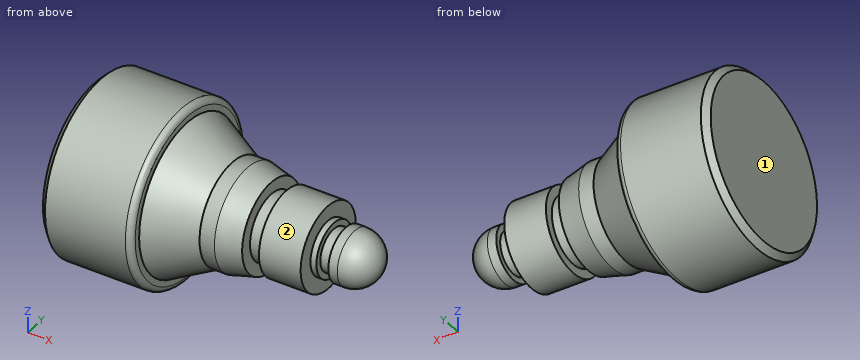
from build123d import *

# Parameters (mm, degrees)
F2_SIZE = 2
F3_R    = 2
F4_R    = 9


with BuildPart() as f1:
    # F0 (on Front) → F1 (revolve)
    with BuildSketch(Plane.XZ):
        Polygon((0, 29), (0, 0), (96, 0), (96, 9), (84, 9), (84, 7), (80, 7), (80, 9), (78, 9), (78, 14), (64, 14), (64, 11), (59, 11), (59, 15), (51, 17), (46, 17), (31, 25), (31, 29), align=None)
    revolve(axis=Axis((48, 0, 0), (1, 0, 0)))

    # F2
    f2_edges = [f1.edges().sort_by_distance(p)[0] for p in [
        (0, 0, -29),
    ]]
    chamfer(f2_edges, length=F2_SIZE)

    # F3
    f3_edges = [f1.edges().sort_by_distance(p)[0] for p in [
        (31, 0, -29),
    ]]
    fillet(f3_edges, radius=F3_R)

    # F4
    f4_edges = [f1.edges().sort_by_distance(p)[0] for p in [
        (96, 0, -9),
    ]]
    fillet(f4_edges, radius=F4_R)


solid = f1.part
Verification items for the finished model (mm, model axes). Face numbers are marked on the shaded views. A direction names the side the tool comes from. Coordinates: 2 decimals unless noted, no trailing zeros. Order: outer loops, then holes, each group sorted by start corner. A loop starts at its lowest first (then second) coordinate and runs counter-clockwise, first axis right, second up. Notation, with made-up numbers: M 18,-28.75 L 28,-28.75 A20 cw 28,6.25 Z; hole C 1.25,36 d1. An arc over 180 degrees is marked long. One line per item, written item: value. Start each with the question number.
Item 1: Access from +Z, -Z, +X, -X, +Y, -Y to the whole of each face (thin tool, end or side, straight path). Record for the marked faces 1 and 2.
Item 2: Scan lines: probe 1 along X at (y, z) = (-10.5, 2.5); probe 2 along Y at (x, z) = (11, 23.5); probe 3 along X at (y, z) = (-25, -8). Record each from-to range of solid material in increasing order.
Item 3: Gauge pin test, flat ends, axial feed: pin 1 (5 mm diameter, centred on y = 19.5, z = -1, fed in from -X); pin 2 (10 mm diameter, centred on x = 73.5, y = -12, fed in from +Z); pin 3 (1 mm diameter, centred on x = 17.5, z = 16.5, fed in from +Y); pin 4 (3 mm diameter, centred on y = -12.5, z = 1, fed in from +X). Record the tip position at first contact, or that the pin passes through.
Item 4: Sectioned sample at A-A (x = 71). Enter the section's corners in (y, z).
Conclusion:
1. face 1: +Z, -Z, -X, +Y, -Y
1. face 2: +X
2. probe 1: x = 0 to 78
2. probe 2: y = -16.99 to 16.99
2. probe 3: x = 0 to 31
3. pin 1: stops at x = 0
3. pin 2: stops at z = 12.12
3. pin 3: stops at y = 24.19
3. pin 4: stops at x = 78
4. outline: C 0,0 d28
